Part print with two shaded views. Sizes in mm from the minimum x, y, z corner. Round coordinates to 2 decimals unless told otherwise and drop trailing zeros. Write each loop counter-clockwise with the first axis right and the second up, starting at its lowest first coordinate (ties: lowest second). Pieces come first, ordered by that corner, then holes. Notation, with made-up numbers: M 28,45 L 35,45 A10 cw 35,61 Z; hole C 29,89 d3. An arc over 180 degrees is marked long. One line per question, with ' | ' between items. Start each with the question number.
1) Wall check: probe 1 along Z at (x, y) = (8, 1); probe 2 along X at (y, z) = (1.3, 32); probe 3 along X at (y, z) = (0.9, 19). Give the ranges that are in metal, low to high. Write a range as [from, to].
2) Saw through at A-A (x = 8). List the corners of the cut face in (y, z), plus the area to 3 significant figures.
3) Saw through at D-D (x = 25). List the corners of the cut face in (y, z).
4) Drop flat-ended pins along their axis: pin 1 Ø4 at (x, z) = (8.5, 33) entering from +Y; pin 2 Ø5 at (x, z) = (27, 19) entering from -Y. Give the stop position or say it passes through.
5) Saw through at C-C (y = 0.5). List the corners of the cut face in (x, z).
6) Saw through at B-B (z = 6). List the corners of the cut face in (x, y), plus the area to 3 significant figures.
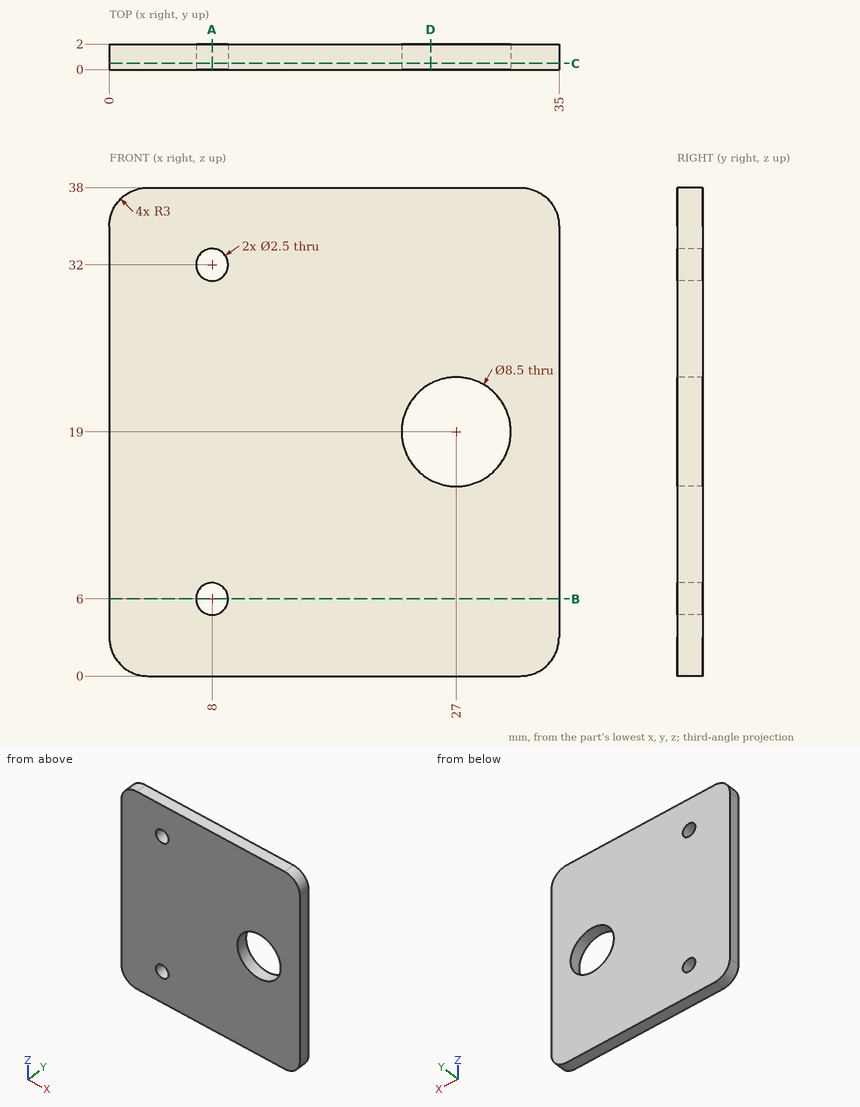
Answer key:
1) probe 1: z = [0, 4.75], [7.25, 30.75], [33.25, 38] | probe 2: x = [0, 6.75], [9.25, 35] | probe 3: x = [0, 22.75], [31.25, 35]
2) outline: M 0,0 L 2,0 L 2,4.75 L 0,4.75 Z; M 0,7.25 L 2,7.25 L 2,30.75 L 0,30.75 Z; M 0,33.25 L 2,33.25 L 2,38 L 0,38 Z | area: 66.0 mm2
3) outline: M 0,0 L 2,0 L 2,15.25 L 0,15.25 Z; M 0,22.75 L 2,22.75 L 2,38 L 0,38 Z
4) pin 1: stops at y = 2 | pin 2: passes through
5) outline: M 0,3 A3 ccw 3,0 L 32,0 A3 ccw 35,3 L 35,35 A3 ccw 32,38 L 3,38 A3 ccw 0,35 Z; hole C 8,6 d2.5; hole C 8,32 d2.5; hole C 27,19 d8.5
6) outline: M 0,0 L 6.75,0 L 6.75,2 L 0,2 Z; M 9.25,0 L 35,0 L 35,2 L 9.25,2 Z | area: 65.0 mm2
